Could you check a few things on this model? Use its own coordinates, in mm. Face numbers are marked on the shaded views. A direction names the side the tool comes from. Round coordinates to 2 decimals unless told otherwise and drop trailing zeros. Order: outer loops, then holes, each group sorted by start corner. A loop starts at its lowest first (then second) coordinate and runs counter-clockwise, first axis right, second up. Notation, with made-up numbers: M -10,-17.5 L 7,-17.5 A19 cw 7,12.5 Z; hole C 64,-11 d6. An arc over 180 degrees is marked long. Write each question's results on one line, items separated by ' | '. Start each with the question number.
1. We'd pull the mould along Z, two halves only. Please class the marked faces 1, 2 and 3: released by +Z, released by -Z, zero draft, split by the parting line, or undercut.
2. For the marked faces 4, 5 and 6, which set-ups out of +Z, -Z, +X, -X, +Y, -Y let a thin tool reach every point of the face, with its end or its side?
3. Please list where these lines run through material, in increasing order: L1, parallel to Y at x = -28, z = -32; L2, parallel to Z at x = -3, y = 44; L3, parallel to Y at x = -10.5, z = 4.5.
4. Suppose I cut it at C-C on y = 12. Write out the boundary of the cut face in (x, z), and give its area (3 significant figures).
5. Suppose I cut it at B-B on x = 31.5. Write out the boundary of the cut face in (y, z).
6. I'm going to push flat-ended pins straight in: pin 1 (1.9 mm diameter, centred on x = 0, z = 35, fed in from -Y); pin 2 (1.9 mm diameter, centred on x = 0, z = -35, fed in from +Y); pin 3 (10 mm diameter, centred on x = 12.5, y = 9.5, fed in from -Z). Where does each tip first touch, or does it pass through?
7. Suppose I cut it at A-A on y = 33. Write out the boundary of the cut face in (x, z), and give its area (3 significant figures).
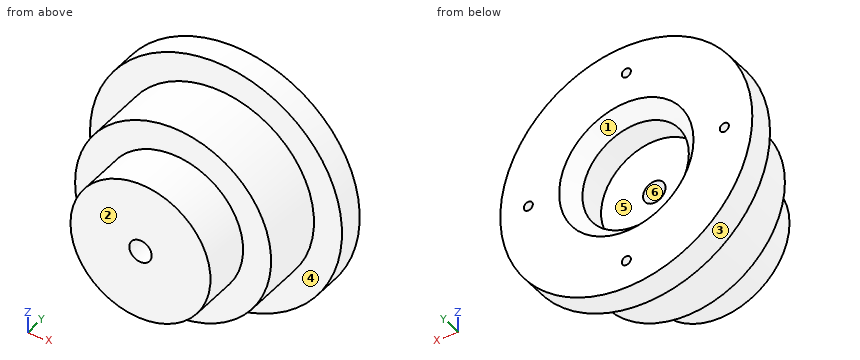
Autodesk Inventor part; units mm, degrees
ref_plane "YZ Plane" through (0, 0, 0) normal (1, 0, 0) x (0, 1, 0)
ref_plane "XZ Plane" through (0, 0, 0) normal (0, 1, 0) x (-1, 0, 0)
ref_plane "XY Plane" through (0, 0, 0) normal (0, 0, 1) x (1, 0, 0)
sketch "Sketch2" plane through (0, 0, 0) normal (0, 0, 1) x (1, 0, 0)
  line L0 (-4, 0) -> (-25, 0)
  line L1 (-25, 0) -> (-25, 17.5)
  line L2 (-25, 17.5) -> (-35, 17.5)
  line L3 (-4, 35) -> (-4, 0)
  line L4 (0, 0) -> (0, 29) construction
  line L5 (-4, 35) -> (-19, 35)
  line L6 (-19, 35) -> (-19, 50)
  line L7 (-35, 17.5) -> (-35, 40.5)
  line L8 (-19, 50) -> (-45, 50)
  line L9 (-45, 50) -> (-45, 40.5)
  line L10 (-45, 40.5) -> (-35, 40.5)
  dimension "d11" = 8
  dimension "d13" = 50
  dimension "d28" = 17.5
  dimension "d29" = 35
  dimension "d30" = 15
  dimension "d34" = 70
  dimension "d35" = 50
  dimension "d36" = 23
  dimension "d37" = 90
revolve "Revolution1" add sketch "Sketch2" angle 360 about axis through (0, 0, 0) along (0, 1, 0)
chamfer "Chamfer1" distance 5 angle 45 1 edges at (19, 50, 0)
sketch "Sketch3" plane through (0, 50, 0) normal (0, 1, 0) x (1, 0, 0)
  point P0 (0, 0)
  point P1 (0, 35)
  dimension "d38" = 35
hole "Hole1" at (0, 50, -35) direction (0, -1, 0) diameter 3.242 depth 8 tip angle 118
pattern_circular "Circular Pattern1" count 4 over 360 about axis through (0, 42.5, 0) along (0, 1, 0) of "Hole1"
properties part number "M17 - Coil Support Part" material "UHMW, Black"
Filled sheet:
1) face 1: undercut | face 2: zero draft | face 3: split by the parting line
2) face 4: -Y | face 5: +Y | face 6: +Y, -Y
3) L1: y = 40.5 to 50 | L2: z = -44.9 to -18.76, 18.76 to 44.9 | L3: y = 0 to 35
4) outline: C 0,0 d50; hole C 0,0 d8 | area: 1,910 mm^2
5) outline: M 17.5,-15.26 L 40.5,-15.26 L 40.5,-32.14 L 50,-32.14 L 50,32.14 L 40.5,32.14 L 40.5,15.26 L 17.5,15.26 Z
6) pin 1: stops at y = 17.5 | pin 2: stops at y = 41.6 | pin 3: stops at z = -23.85
7) outline: C 0,0 d70; hole C 0,0 d8 | area: 3,800 mm^2
